Design review of the part built by this model. Coordinates are the model's own, in mm. A direction names the side the tool comes from. Round coordinates to 2 decimals unless told otherwise and drop trailing zeros. Loops run counter-clockwise (first coordinate to the right, second up) from the corner with the lowest first, then second, coordinate; pieces in that order, holes last. Notation, with made-up numbers: (10, -36.5) -> (62, -36.5) arc R26 cw to (62, 2.5) -> close; hole circle Ø7 at (4, -2.75). An arc over 180 degrees is marked (long way). Write each question's results on one line, items separated by ' | '. Start each with the question number.
from build123d import *

# Parameters (mm, degrees)
BOSS_EXTRUDE1_DEPTH = 4
SKETCH2_W           = 2.5
SKETCH2_H           = 4
CUT_EXTRUDE1_DEPTH  = 4


with BuildPart() as part:
    # Sketch1 → Boss-Extrude1 (new body)
    with BuildSketch(Plane.XY):
        with BuildLine():
            Line((0, 0), (10, 0))
            Line((10, 0), (10, 4))
            Line((10, 4), (12.5, 4))
            Line((12.5, 4), (12.5, 8))
            Line((12.5, 8), (10, 8))
            Line((10, 8), (10, 12))
            Line((10, 12), (15, 12))
            Line((15, 12), (15, 17))
            ThreePointArc((15, 17), (5, 27), (-5, 17))
            Line((-5, 17), (-5, 12))
            Line((-5, 12), (0, 12))
            Line((0, 12), (0, 8))
            Line((0, 8), (-2.5, 8))
            Line((-2.5, 8), (-2.5, 4))
            Line((-2.5, 4), (0, 4))
            Line((0, 4), (0, 0))
        make_face()
        Polygon((3.354551733, 18.071172359), (6.645448267, 18.071172359), (8.290896534, 20.921172359), (6.645448267, 23.771172359), (3.354551733, 23.771172359), (1.709103466, 20.921172359), align=None, mode=Mode.SUBTRACT)
        Polygon((8.290896534, 10.5), (6.645448267, 13.35), (3.354551733, 13.35), (1.709103466, 10.5), (3.354551733, 7.65), (6.645448267, 7.65), align=None, mode=Mode.SUBTRACT)
    extrude(amount=BOSS_EXTRUDE1_DEPTH)

    # Sketch2 → Cut-Extrude1 (cut)
    with BuildSketch(Plane.XY.offset(4)):
        with Locations((-1.25, 6)):
            Rectangle(SKETCH2_W, SKETCH2_H)
        with Locations((11.25, 6)):
            Rectangle(SKETCH2_W, SKETCH2_H)
    extrude(amount=-CUT_EXTRUDE1_DEPTH, mode=Mode.SUBTRACT)


solid = part.part
1) Take a section at C-C (y = 12.75). Write out the cut boundary in (x, z).
2) The part is to be moulded in two halves that separate along X. For faces 6 (the face through (10, 6, 2)), 7 (the face through (2.52, 9.095, 1.972)), 8 (the face through (2.543, 22.366, 1.972)), 9 (the face through (5, 14, 4)), say which applies: +X half, -X half, draft (parallel to the pull), parting line (faces both ways), or undercut.
3) For faces 1 (the face through (5, 27, 2)), 2 (the face through (5, 14, 0)), 3 (the face through (5, 23.771, 2)), 4 (the face through (-3, 12, 2)), 5 (the face through (12, 12, 2)), list the 3-axis set-ups (+Z, -Z, +X, -X, +Y, -Y) from which the entire face can be reached by the end or side of a thin tool; tool diameter is ignored.
4) Take a section at B-B (z = 1.05). Write out the cut boundary in (x, y), plus the area to 3 significant figures.
5) Take a section at A-A (x = 5). Write out the cut boundary in (y, z).
6) Take a section at D-D (y = 4.75). Write out the cut boundary in (x, z).
7) Insertion check: pin 1 (1.5 mm diameter, centred on y = 6.5, z = 1.5, fed in from -X); pin 2 (1.5 mm diameter, centred on y = 7.5, z = 2.5, fed in from +X); pin 3 (2 mm diameter, centred on x = 13.5, z = 2, fed in from -Y). Each pin has a flat end and moves straight along its axis. Give the tip position at first contact, or say it passes through.
8) To check wall thickness, follow line 1 (Y direction, x = 5.25, z = 1.4); line 2 (Y direction, x = 2, z = 1.85); line 3 (X direction, y = 13, z = 2.6). State the ranges of each line that lie inside material, in increasing order. Write a range as from..to.
Geometry check:
1) outline: (-5, 0) -> (3.01, 0) -> (3.01, 4) -> (-5, 4) -> close; (6.99, 0) -> (15, 0) -> (15, 4) -> (6.99, 4) -> close
2) face 6: +X half | face 7: undercut | face 8: undercut | face 9: draft
3) face 1: +Z, -Z, +Y | face 2: -Z, +X, -X, +Y, -Y | face 3: +Z, -Z | face 4: +Z, -Z, -X, -Y | face 5: +Z, -Z, +X, -Y
4) outline: (-5, 12) -> (0, 12) -> (0, 0) -> (10, 0) -> (10, 12) -> (15, 12) -> (15, 17) arc R10 ccw to (-5, 17) -> close; hole (1.71, 10.5) -> (3.35, 7.65) -> (6.65, 7.65) -> (8.29, 10.5) -> (6.65, 13.35) -> (3.35, 13.35) -> close; hole (1.71, 20.92) -> (3.35, 18.07) -> (6.65, 18.07) -> (8.29, 20.92) -> (6.65, 23.77) -> (3.35, 23.77) -> close | area: 321 mm^2
5) outline: (0, 0) -> (7.65, 0) -> (7.65, 4) -> (0, 4) -> close; (13.35, 0) -> (18.07, 0) -> (18.07, 4) -> (13.35, 4) -> close; (23.77, 0) -> (27, 0) -> (27, 4) -> (23.77, 4) -> close
6) outline: (0, 0) -> (10, 0) -> (10, 4) -> (0, 4) -> close
7) pin 1: stops at x = 0 | pin 2: stops at x = 10 | pin 3: stops at y = 12
8) line 1: y = 0..7.65, 13.35..18.07, 23.77..27 | line 2: y = 0..10, 11..20.42, 21.43..26.54 | line 3: x = -5..3.15, 6.85..15
